The model under review builds one solid part; all positions refer to its coordinate system, in mm. Face numbers are marked on the shaded views. A direction names the side the tool comes from. Coordinates: 2 decimals unless noted, no trailing zeros. Order: outer loops, then holes, each group sorted by start corner. A loop starts at its lowest first (then second) coordinate and runs counter-clockwise, first axis right, second up.
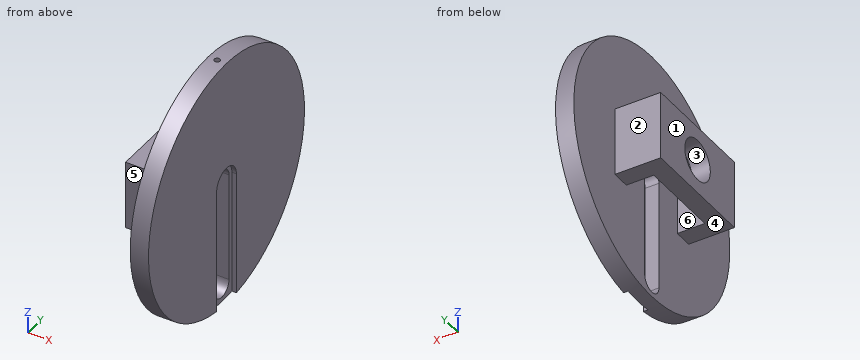
```python
from build123d import *

# Parameters (mm, degrees)
SKETCH_1_R             = 7.5
EXTRUDE_1_DEPTH        = 10
SKETCH_5_W             = 30
SKETCH_5_H             = 52
EXTRUDE_2_DEPTH        = 8
SKETCH_6_W             = 30
SKETCH_6_H             = 8
EXTRUDE_3_DEPTH        = 12
SKETCH_7_R             = 55
EXTRUDE_4_DEPTH        = 8
CUT_EXTRUDE_4_REACH    = 40
CUT_EXTRUDE_6_DEPTH    = 2
CUT_EXTRUDE_7_REACH    = 40
SKETCH_12_R            = 9
HOLE_WIZARD_M3_1_D     = 2.5
HOLE_WIZARD_M3_1_DEPTH = 5
HOLE_WIZARD_M3_1_TIP   = 0.751075774


with BuildPart() as part:
    # 草图1 → 凸台-拉伸1 (new body)
    with BuildSketch(Plane(origin=(0, 0, 0), x_dir=(0, 0, -1), z_dir=(1, 0, 0))):
        Circle(SKETCH_1_R)
    extrude(amount=EXTRUDE_1_DEPTH)

    # 草图5 → 凸台-拉伸2 (add)
    with BuildSketch(Plane(origin=(10, 0, 0), x_dir=(0, 0, -1), z_dir=(1, 0, 0))):
        Rectangle(SKETCH_5_W, SKETCH_5_H)
    extrude(amount=EXTRUDE_2_DEPTH)

    # 草图6 → 凸台-拉伸3 (add)
    with BuildSketch(Plane(origin=(18, 0, 0), x_dir=(0, 0, -1), z_dir=(1, 0, 0))):
        with Locations((0, 22)):
            Rectangle(SKETCH_6_W, SKETCH_6_H)
        with Locations((0, -22)):
            Rectangle(SKETCH_6_W, SKETCH_6_H)
    extrude(amount=EXTRUDE_3_DEPTH)

    # 草图7 → 凸台-拉伸4 (add)
    with BuildSketch(Plane(origin=(30, 0, 0), x_dir=(0, 0, -1), z_dir=(1, 0, 0))):
        Circle(SKETCH_7_R)
    extrude(amount=EXTRUDE_4_DEPTH)

    # 草图8 → 切除-拉伸4 (cut, up to next)
    with BuildSketch(Plane(origin=(38, 0, 0), x_dir=(0, 0, -1), z_dir=(1, 0, 0)), mode=Mode.PRIVATE) as cut_extrude_4_sk1:
        with BuildLine():
            Line((0, 5), (48, 5))
            ThreePointArc((48, 5), (53, 0), (48, -5))
            Line((48, -5), (0, -5))
            ThreePointArc((0, -5), (-5, 0), (0, 5))
        make_face()
    cut_extrude_4_tool1 = extrude(cut_extrude_4_sk1.sketch, amount=-CUT_EXTRUDE_4_REACH, mode=Mode.PRIVATE) & part.part
    add(cut_extrude_4_tool1.solids().sort_by_distance((38, 0, -24))[0], mode=Mode.SUBTRACT)

    # 草图11 → 切除-拉伸6 (cut)
    with BuildSketch(Plane(origin=(38, 0, 0), x_dir=(0, 0, -1), z_dir=(1, 0, 0))):
        with BuildLine():
            Line((0, 7), (54.552726788, 7))
            ThreePointArc((54.552726788, 7), (55, 0), (54.552726788, -7))
            Line((54.552726788, -7), (0, -7))
            ThreePointArc((0, -7), (-7, 0), (0, 7))
        make_face()
    extrude(amount=-CUT_EXTRUDE_6_DEPTH, mode=Mode.SUBTRACT)

    # 草图12 → 切除-拉伸7 (cut, up to next)
    with BuildSketch(Plane.ZY, mode=Mode.PRIVATE) as cut_extrude_7_sk1:
        Circle(SKETCH_12_R)
    cut_extrude_7_tool1 = extrude(cut_extrude_7_sk1.sketch, amount=-CUT_EXTRUDE_7_REACH, mode=Mode.PRIVATE) & part.part
    add(cut_extrude_7_tool1.solids().sort_by_distance((0, 0, 0))[0], mode=Mode.SUBTRACT)

    # M3 螺纹孔1
    with Locations(Plane(origin=(33.918718573, 0, 55), x_dir=(1, 0, 0), z_dir=(0, 0, 1))):
        with Locations((0, 0)):
            Hole(HOLE_WIZARD_M3_1_D / 2, depth=HOLE_WIZARD_M3_1_DEPTH)
            with Locations((0, 0, -(HOLE_WIZARD_M3_1_DEPTH + HOLE_WIZARD_M3_1_TIP / 2))):  # 118° drill point
                Cone(0, HOLE_WIZARD_M3_1_D / 2, HOLE_WIZARD_M3_1_TIP, mode=Mode.SUBTRACT)


solid = part.part
```
(1) We need section C-C, the plane y = -20. Write out the cut boundary in (x, z), and give its area (3 significant figures).
A:
outline: (10, -15) - (30, -15) - (30, -51.23) - (38, -51.23) - (38, 51.23) - (30, 51.23) - (30, 15) - (10, 15) - close
area: 1,420 mm2
(2) For pin 1 Ø6.5 at (x, z) = (31.5, -32) entering from +Y; pin 2 Ø10 at (x, z) = (24.5, -3.5) entering from -Y; pin 3 Ø9.5 at (x, z) = (22.5, 1) entering from +Y, all flat-tipped, find the tip position at first contact; note any pin that passes through.
A:
pin 1: stops at y = 46.89
pin 2: stops at y = -26
pin 3: stops at y = 26
(3) We need section B-B, the plane z = -4. Write out the cut boundary in (x, y), and give its area (3 significant figures).
A:
outline: (10, -26) - (30, -26) - (30, -54.85) - (38, -54.85) - (38, -7) - (36, -7) - (36, -5) - (30, -5) - (30, -18) - (18, -18) - (18, -8.06) - (10, -8.06) - close; (10, 8.06) - (18, 8.06) - (18, 18) - (30, 18) - (30, 5) - (36, 5) - (36, 7) - (38, 7) - (38, 54.85) - (30, 54.85) - (30, 26) - (10, 26) - close
area: 1,270 mm2
(4) Machinability: for the marked faces 1, 2 and 3, which of the approach directions +Z, -Z, +X, -X, +Y, -Y give a long, thin tool a straight path to every point of the face, cutting with its end or side? Answer none if there is none.
A:
face 1: +Z, -Z, -X, +Y, -Y
face 2: +Z, -Z, -X, +Y
face 3: -X
(5) We need section A-A, the plane x = 14. Write out the cut boundary in (y, z).
A:
outline: (-26, -15) - (26, -15) - (26, 15) - (-26, 15) - close; hole circle Ø18 at (0, 0)
(6) Draft analysis for pull direction Y (two halves, no side actions). For the marked faces 4, 5 and 6, state which applies: released by +Y, released by -Y, zero draft, split by the parting line, or undercut.
A:
face 4: zero draft
face 5: released by -Y
face 6: undercut
(7) We need section D-D, the plane z = 19. Write out the cut boundary in (x, y).
A:
outline: (30, -51.61) - (38, -51.61) - (38, 51.61) - (30, 51.61) - close
(8) Wall thickness on probe 1 along Y at (x, z) = (27.75, 10); probe 2 along Y at (x, z) = (13.25, 0); probe 3 along X at (y, z) = (-5, 11): over which ranges is each line inside the solid? List them lowest first.
A:
probe 1: y = -26 to -18, 18 to 26
probe 2: y = -26 to -9, 9 to 26
probe 3: x = 10 to 18, 30 to 38
